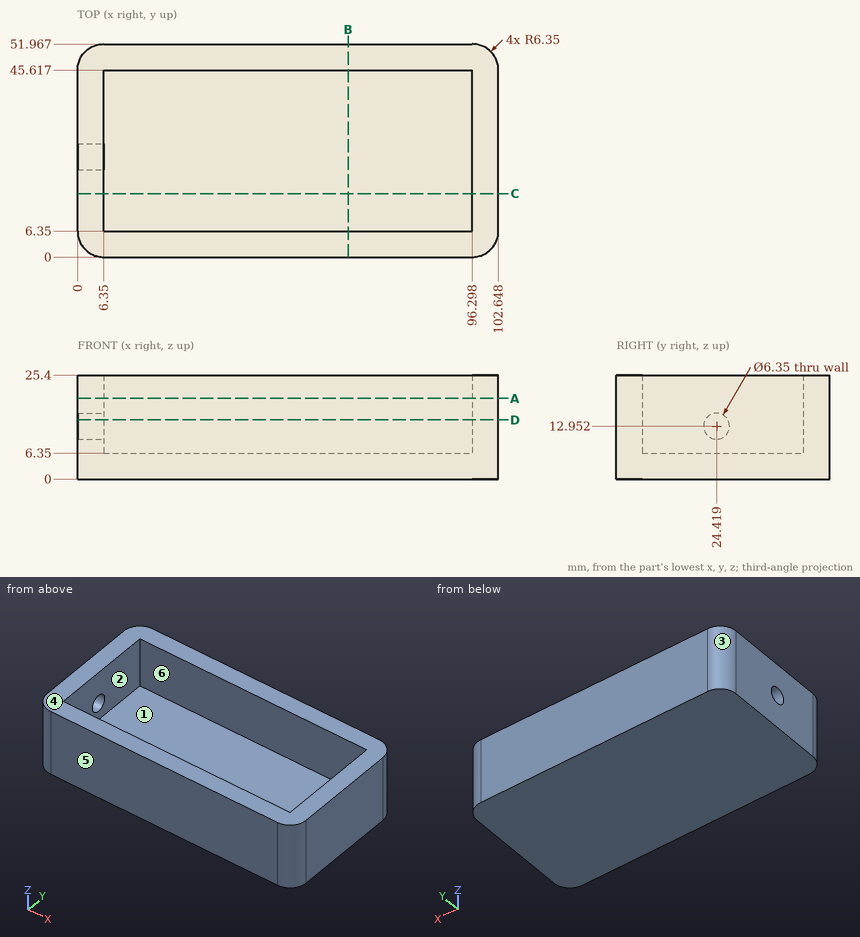
Design review of the part shown in the three views and the two pictorial views. Dimensions are in mm from the part's minimum x, y and z. A direction names the side the tool comes from. Round coordinates to 2 decimals unless told otherwise and drop trailing zeros. Write each loop counter-clockwise with the first axis right and the second up, starting at its lowest first coordinate (ties: lowest second). Pieces come first, ordered by that corner, then holes.
1) Take a section at B-B on x = 66. Give the boundary of the cut face in (y, z).
Answer below:
outline: (0, 0) - (51.97, 0) - (51.97, 25.4) - (45.62, 25.4) - (45.62, 6.35) - (6.35, 6.35) - (6.35, 25.4) - (0, 25.4) - close
2) Take a section at C-C on y = 15.5. Give the boundary of the cut face in (x, z).
Answer below:
outline: (0, 0) - (102.65, 0) - (102.65, 25.4) - (96.3, 25.4) - (96.3, 6.35) - (6.35, 6.35) - (6.35, 25.4) - (0, 25.4) - close
3) Mouldability with a two-part tool opening along Y and no side actions: class the marked faces 1, 2, 3 and 4 as +Y half, -Y half, draft (parallel to the pull), parting line (faces both ways), or undercut.
Answer below:
face 1: undercut
face 2: undercut
face 3: +Y half
face 4: draft
4) Insertion check: pin 1 Ø15 at (x, z) = (46.5, 13) entering from -Y; pin 2 Ø1 at (x, y) = (59, 7.5) entering from +Z; pin 3 Ø5.5 at (y, z) = (24.42, 12.95) entering from -X. Each pin has a flat end and moves straight along its axis. Give the tip position at first contact, or say it passes through.
Answer below:
pin 1: stops at y = 0
pin 2: stops at z = 6.35
pin 3: stops at x = 96.3
5) Machinability: for the marked faces 5 and 6, which of the approach directions +Z, -Z, +X, -X, +Y, -Y give a long, thin tool a straight path to every point of the face, cutting with its end or side? Answer none if there is none.
Answer below:
face 5: +Z, -Z, +X, -X, -Y
face 6: +Z
6) Take a section at D-D on z = 14.5. Give the boundary of the cut face in (x, y), then the cut area to 3 significant figures.
Answer below:
outline: (0, 6.35) arc R6.35 ccw to (6.35, 0) - (96.3, 0) arc R6.35 ccw to (102.65, 6.35) - (102.65, 45.62) arc R6.35 ccw to (96.3, 51.97) - (6.35, 51.97) arc R6.35 ccw to (0, 45.62) - (0, 27.19) - (6.35, 27.19) - (6.35, 45.62) - (96.3, 45.62) - (96.3, 6.35) - (6.35, 6.35) - (6.35, 21.65) - (0, 21.65) - close
area: 1,730 mm2
7) For line 1 along Y through (x, z) = (80, 10.25); line 2 along X through (y, z) = (34.5, 7); line 3 along Z through (x, y) = (90.5, 45.5), list the stretches that pass through material, from the lowest coordinate up.
Answer below:
line 1: y = 0 to 6.35, 45.62 to 51.97
line 2: x = 0 to 6.35, 96.3 to 102.65
line 3: z = 0 to 6.35
8) Take a section at A-A on z = 19.75. Give the boundary of the cut face in (x, y).
Answer below:
outline: (0, 6.35) arc R6.35 ccw to (6.35, 0) - (96.3, 0) arc R6.35 ccw to (102.65, 6.35) - (102.65, 45.62) arc R6.35 ccw to (96.3, 51.97) - (6.35, 51.97) arc R6.35 ccw to (0, 45.62) - close; hole (6.35, 6.35) - (96.3, 6.35) - (96.3, 45.62) - (6.35, 45.62) - close
